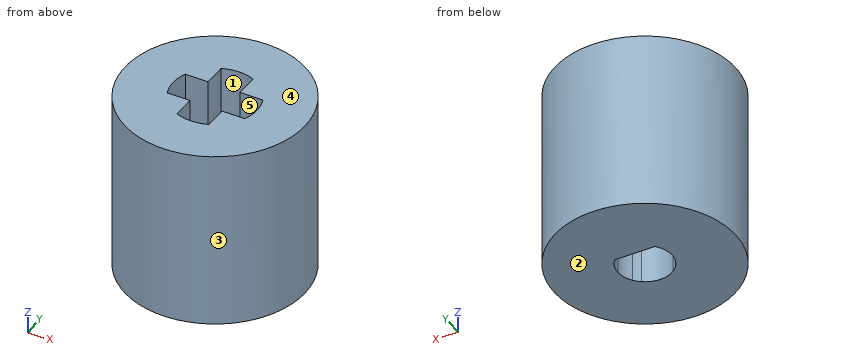
from build123d import *

# Parameters (mm, degrees)
SKETCH1_R           = 5
SKETCH1_R_2         = 2.34
BOSS_EXTRUDE1_DEPTH = 5
BOSS_EXTRUDE2_START = -5
SKETCH1_3_R         = 5
SKETCH1_3_R_2       = 2.34
BOSS_EXTRUDE2_DEPTH = 5


with BuildPart() as part:
    # Sketch1 → Boss-Extrude1 (new body)
    # profile 1 of 11: a face of its own
    with BuildSketch(Plane.XY):
        Circle(SKETCH1_R)
        Circle(SKETCH1_R_2, mode=Mode.SUBTRACT)
    # profile 2 of 11: a face of its own
    with BuildSketch(Plane.XY):
        with BuildLine():
            Line((-0.89, 1.207435298), (-0.89, 2.164139552))
            ThreePointArc((-0.89, 2.164139552), (-1.654629868, 1.654629868), (-2.164139552, 0.89))
            Line((-2.164139552, 0.89), (-1.207435298, 0.89))
            ThreePointArc((-1.207435298, 0.89), (-1.164034729, 0.946056631), (-1.118033989, 1))
            ThreePointArc((-1.118033989, 1), (-1.009359934, 1.109591152), (-0.89, 1.207435298))
        make_face()
    # profile 3 of 11: a face of its own
    with BuildSketch(Plane.XY):
        with BuildLine():
            ThreePointArc((2.164139552, 0.89), (1.654629868, 1.654629868), (0.89, 2.164139552))
            Line((0.89, 2.164139552), (0.89, 1.207435298))
            ThreePointArc((0.89, 1.207435298), (1.009359934, 1.109591152), (1.118033989, 1))
            ThreePointArc((1.118033989, 1), (1.164034729, 0.946056631), (1.207435298, 0.89))
            Line((1.207435298, 0.89), (2.164139552, 0.89))
        make_face()
    # profile 4 of 11: a face of its own
    with BuildSketch(Plane.XY):
        with BuildLine():
            Line((-0.89, 0.89), (-0.89, 1))
            Line((-0.89, 1), (-1.118033989, 1))
            ThreePointArc((-1.118033989, 1), (-1.164034729, 0.946056631), (-1.207435298, 0.89))
            Line((-1.207435298, 0.89), (-0.89, 0.89))
        make_face()
    # profile 5 of 11: a face of its own
    with BuildSketch(Plane.XY):
        with BuildLine():
            Line((-0.89, 1), (-0.89, 1.207435298))
            ThreePointArc((-0.89, 1.207435298), (-1.009359934, 1.109591152), (-1.118033989, 1))
            Line((-1.118033989, 1), (-0.89, 1))
        make_face()
    # profile 6 of 11: a face of its own
    with BuildSketch(Plane.XY):
        with BuildLine():
            ThreePointArc((1.118033989, 1), (1.009359934, 1.109591152), (0.89, 1.207435298))
            Line((0.89, 1.207435298), (0.89, 1))
            Line((0.89, 1), (1.118033989, 1))
        make_face()
    # profile 7 of 11: a face of its own
    with BuildSketch(Plane.XY):
        with BuildLine():
            Line((1.118033989, 1), (0.89, 1))
            Line((0.89, 1), (0.89, 0.89))
            Line((0.89, 0.89), (1.207435298, 0.89))
            ThreePointArc((1.207435298, 0.89), (1.164034729, 0.946056631), (1.118033989, 1))
        make_face()
    # profile 8 of 11: a face of its own
    with BuildSketch(Plane.XY):
        with BuildLine():
            Line((1.207435298, -0.89), (0.89, -0.89))
            Line((0.89, -0.89), (0.89, -1.207435298))
            ThreePointArc((0.89, -1.207435298), (1.060660172, -1.060660172), (1.207435298, -0.89))
        make_face()
    # profile 9 of 11: a face of its own
    with BuildSketch(Plane.XY):
        with BuildLine():
            ThreePointArc((0.89, -2.164139552), (1.654629868, -1.654629868), (2.164139552, -0.89))
            Line((2.164139552, -0.89), (1.207435298, -0.89))
            ThreePointArc((1.207435298, -0.89), (1.060660172, -1.060660172), (0.89, -1.207435298))
            Line((0.89, -1.207435298), (0.89, -2.164139552))
        make_face()
    # profile 10 of 11: a face of its own
    with BuildSketch(Plane.XY):
        with BuildLine():
            Line((-1.207435298, -0.89), (-2.164139552, -0.89))
            ThreePointArc((-2.164139552, -0.89), (-1.654629868, -1.654629868), (-0.89, -2.164139552))
            Line((-0.89, -2.164139552), (-0.89, -1.207435298))
            ThreePointArc((-0.89, -1.207435298), (-1.060660172, -1.060660172), (-1.207435298, -0.89))
        make_face()
    # profile 11 of 11: a face of its own
    with BuildSketch(Plane.XY):
        with BuildLine():
            Line((-0.89, -0.89), (-1.207435298, -0.89))
            ThreePointArc((-1.207435298, -0.89), (-1.060660172, -1.060660172), (-0.89, -1.207435298))
            Line((-0.89, -1.207435298), (-0.89, -0.89))
        make_face()
    extrude(amount=BOSS_EXTRUDE1_DEPTH)

    # Sketch1_3 → Boss-Extrude2 (add)
    # profile 1 of 16: a face of its own
    with BuildSketch(Plane.XY.offset(BOSS_EXTRUDE2_START)):
        Circle(SKETCH1_3_R)
        Circle(SKETCH1_3_R_2, mode=Mode.SUBTRACT)
    # profile 2 of 16: a face of its own
    with BuildSketch(Plane.XY.offset(BOSS_EXTRUDE2_START)):
        with BuildLine():
            ThreePointArc((0.89, -2.164139552), (1.654629868, -1.654629868), (2.164139552, -0.89))
            Line((2.164139552, -0.89), (1.207435298, -0.89))
            ThreePointArc((1.207435298, -0.89), (1.060660172, -1.060660172), (0.89, -1.207435298))
            Line((0.89, -1.207435298), (0.89, -2.164139552))
        make_face()
    # profile 3 of 16: a face of its own
    with BuildSketch(Plane.XY.offset(BOSS_EXTRUDE2_START)):
        with BuildLine():
            Line((-1.207435298, 0.89), (-2.164139552, 0.89))
            ThreePointArc((-2.164139552, 0.89), (-2.34, 0), (-2.164139552, -0.89))
            Line((-2.164139552, -0.89), (-1.207435298, -0.89))
            ThreePointArc((-1.207435298, -0.89), (-1.5, 0), (-1.207435298, 0.89))
        make_face()
    # profile 4 of 16: a face of its own
    with BuildSketch(Plane.XY.offset(BOSS_EXTRUDE2_START)):
        with BuildLine():
            ThreePointArc((2.34, 0), (2.295613921, 0.453604149), (2.164139552, 0.89))
            Line((2.164139552, 0.89), (1.207435298, 0.89))
            ThreePointArc((1.207435298, 0.89), (1.424982973, 0.46842665), (1.5, 0))
            ThreePointArc((1.5, 0), (1.424982973, -0.46842665), (1.207435298, -0.89))
            Line((1.207435298, -0.89), (2.164139552, -0.89))
            ThreePointArc((2.164139552, -0.89), (2.295613921, -0.453604149), (2.34, 0))
        make_face()
    # profile 5 of 16: a face of its own
    with BuildSketch(Plane.XY.offset(BOSS_EXTRUDE2_START)):
        with BuildLine():
            ThreePointArc((2.164139552, 0.89), (1.654629868, 1.654629868), (0.89, 2.164139552))
            Line((0.89, 2.164139552), (0.89, 1.207435298))
            ThreePointArc((0.89, 1.207435298), (1.009359934, 1.109591152), (1.118033989, 1))
            ThreePointArc((1.118033989, 1), (1.164034729, 0.946056631), (1.207435298, 0.89))
            Line((1.207435298, 0.89), (2.164139552, 0.89))
        make_face()
    # profile 6 of 16: a face of its own
    with BuildSketch(Plane.XY.offset(BOSS_EXTRUDE2_START)):
        with BuildLine():
            ThreePointArc((0.89, 2.164139552), (0, 2.34), (-0.89, 2.164139552))
            Line((-0.89, 2.164139552), (-0.89, 1.207435298))
            ThreePointArc((-0.89, 1.207435298), (0, 1.5), (0.89, 1.207435298))
            Line((0.89, 1.207435298), (0.89, 2.164139552))
        make_face()
    # profile 7 of 16: a face of its own
    with BuildSketch(Plane.XY.offset(BOSS_EXTRUDE2_START)):
        with BuildLine():
            Line((-0.89, -1.207435298), (-0.89, -2.164139552))
            ThreePointArc((-0.89, -2.164139552), (0, -2.34), (0.89, -2.164139552))
            Line((0.89, -2.164139552), (0.89, -1.207435298))
            ThreePointArc((0.89, -1.207435298), (0, -1.5), (-0.89, -1.207435298))
        make_face()
    # profile 8 of 16: a face of its own
    with BuildSketch(Plane.XY.offset(BOSS_EXTRUDE2_START)):
        with BuildLine():
            Line((-0.89, 1.207435298), (-0.89, 2.164139552))
            ThreePointArc((-0.89, 2.164139552), (-1.654629868, 1.654629868), (-2.164139552, 0.89))
            Line((-2.164139552, 0.89), (-1.207435298, 0.89))
            ThreePointArc((-1.207435298, 0.89), (-1.164034729, 0.946056631), (-1.118033989, 1))
            ThreePointArc((-1.118033989, 1), (-1.009359934, 1.109591152), (-0.89, 1.207435298))
        make_face()
    # profile 9 of 16: a face of its own
    with BuildSketch(Plane.XY.offset(BOSS_EXTRUDE2_START)):
        with BuildLine():
            Line((-1.207435298, 0.89), (-2.164139552, 0.89))
            ThreePointArc((-2.164139552, 0.89), (-2.34, 0), (-2.164139552, -0.89))
            Line((-2.164139552, -0.89), (-1.207435298, -0.89))
            ThreePointArc((-1.207435298, -0.89), (-1.5, 0), (-1.207435298, 0.89))
        make_face()
    # profile 10 of 16: a face of its own
    with BuildSketch(Plane.XY.offset(BOSS_EXTRUDE2_START)):
        with BuildLine():
            ThreePointArc((2.34, 0), (2.295613921, 0.453604149), (2.164139552, 0.89))
            Line((2.164139552, 0.89), (1.207435298, 0.89))
            ThreePointArc((1.207435298, 0.89), (1.424982973, 0.46842665), (1.5, 0))
            ThreePointArc((1.5, 0), (1.424982973, -0.46842665), (1.207435298, -0.89))
            Line((1.207435298, -0.89), (2.164139552, -0.89))
            ThreePointArc((2.164139552, -0.89), (2.295613921, -0.453604149), (2.34, 0))
        make_face()
    # profile 11 of 16: a face of its own
    with BuildSketch(Plane.XY.offset(BOSS_EXTRUDE2_START)):
        with BuildLine():
            Line((-1.207435298, -0.89), (-2.164139552, -0.89))
            ThreePointArc((-2.164139552, -0.89), (-1.654629868, -1.654629868), (-0.89, -2.164139552))
            Line((-0.89, -2.164139552), (-0.89, -1.207435298))
            ThreePointArc((-0.89, -1.207435298), (-1.060660172, -1.060660172), (-1.207435298, -0.89))
        make_face()
    # profile 12 of 16: a face of its own
    with BuildSketch(Plane.XY.offset(BOSS_EXTRUDE2_START)):
        with BuildLine():
            ThreePointArc((1.118033989, 1), (1.009359934, 1.109591152), (0.89, 1.207435298))
            Line((0.89, 1.207435298), (0.89, 1))
            Line((0.89, 1), (1.118033989, 1))
        make_face()
    # profile 13 of 16: a face of its own
    with BuildSketch(Plane.XY.offset(BOSS_EXTRUDE2_START)):
        with BuildLine():
            ThreePointArc((0.89, 1.207435298), (0, 1.5), (-0.89, 1.207435298))
            Line((-0.89, 1.207435298), (-0.89, 1))
            Line((-0.89, 1), (0.89, 1))
            Line((0.89, 1), (0.89, 1.207435298))
        make_face()
    # profile 14 of 16: a face of its own
    with BuildSketch(Plane.XY.offset(BOSS_EXTRUDE2_START)):
        with BuildLine():
            Line((-0.89, 1), (-0.89, 1.207435298))
            ThreePointArc((-0.89, 1.207435298), (-1.009359934, 1.109591152), (-1.118033989, 1))
            Line((-1.118033989, 1), (-0.89, 1))
        make_face()
    # profile 15 of 16: a face of its own
    with BuildSketch(Plane.XY.offset(BOSS_EXTRUDE2_START)):
        with BuildLine():
            ThreePointArc((0.89, 2.164139552), (0, 2.34), (-0.89, 2.164139552))
            Line((-0.89, 2.164139552), (-0.89, 1.207435298))
            ThreePointArc((-0.89, 1.207435298), (0, 1.5), (0.89, 1.207435298))
            Line((0.89, 1.207435298), (0.89, 2.164139552))
        make_face()
    # profile 16 of 16: a face of its own
    with BuildSketch(Plane.XY.offset(BOSS_EXTRUDE2_START)):
        with BuildLine():
            Line((-0.89, -1.207435298), (-0.89, -2.164139552))
            ThreePointArc((-0.89, -2.164139552), (0, -2.34), (0.89, -2.164139552))
            Line((0.89, -2.164139552), (0.89, -1.207435298))
            ThreePointArc((0.89, -1.207435298), (0, -1.5), (-0.89, -1.207435298))
        make_face()
    extrude(amount=BOSS_EXTRUDE2_DEPTH)


solid = part.part
Could you check a few things on this model? Use its own coordinates, in mm. Face numbers are marked on the shaded views. A direction names the side the tool comes from. Give positions to 0.01 mm unless a question says otherwise; leave off trailing zeros. Order: outer loops, then holes, each group sorted by start corner. A loop starts at its lowest first (then second) coordinate and runs counter-clockwise, first axis right, second up.
Item 1: If we section it at A-A, the plane x = 0: Write out the boundary of the cut face in (y, z), plus the area to 3 significant figures.
Item 2: I need wall thicknesses on line 1 (X direction, y = -1.75, z = 2.25); line 2 (Y direction, x = -0.75, z = -0.5); line 3 (Y direction, x = -2, z = 4.25). Which ranges of each line are inside material? Lowest first, please.
Item 3: For the marked faces 1 and 2, which set-ups out of +Z, -Z, +X, -X, +Y, -Y let a thin tool reach every point of the face, with its end or its side?
Item 4: If we mould it in two halves opening along Y, with no side actions, what happens to the marked faces 3, 4 and 5? For each: pulls with the +Y half, pulls with the -Y half, needs draft (parallel to the pull), parting line crosses it, or undercut.
Item 5: If we section it at C-C, the plane y = 0.75: Write out the boundary of the cut face in (x, z), plus the area to 3 significant figures.
Item 6: If we section it at D-D, the plane x = 1.75: Write out the boundary of the cut face in (y, z).
Item 7: I'm going to push flat-ended pins straight in: pin 1 (1.4 mm diameter, centred on x = -1, z = 3, fed in from -Y); pin 2 (6 mm diameter, centred on x = -3.5, z = -1.5, fed in from +Y); pin 3 (0.6 mm diameter, centred on x = 2, y = 0, fed in from +Z). Where does each tip first touch, or does it pass through?
Item 8: If we section it at B-B, the plane z = 0.75: Write out the boundary of the cut face in (x, y), plus the area to 3 significant figures.
Values:
1. outline: (-5, -5) - (-1.5, -5) - (-1.5, 0) - (-2.34, 0) - (-2.34, 5) - (-5, 5) - close; (1, -5) - (5, -5) - (5, 5) - (2.34, 5) - (2.34, 0) - (1, 0) - close
1. area: 64.1 mm2
2. line 1: x = -4.68 to -0.89, 0.89 to 4.68
2. line 2: y = -4.94 to -1.3, 1 to 4.94
2. line 3: y = -4.58 to -0.89, 0.89 to 4.58
3. face 1: +Z
3. face 2: -Z, +X, -X, +Y, -Y
4. face 3: parting line crosses it
4. face 4: needs draft
4. face 5: undercut
5. outline: (-4.94, -5) - (-1.3, -5) - (-1.3, 0) - (-2.22, 0) - (-2.22, 5) - (-4.94, 5) - close; (1.3, -5) - (4.94, -5) - (4.94, 5) - (2.22, 5) - (2.22, 0) - (1.3, 0) - close
5. area: 63.7 mm2
6. outline: (-4.68, -5) - (4.68, -5) - (4.68, 5) - (0.89, 5) - (0.89, 0) - (-0.89, 0) - (-0.89, 5) - (-4.68, 5) - close
7. pin 1: stops at y = -4.99
7. pin 2: stops at y = 4.97
7. pin 3: stops at z = 0
8. outline: circle Ø10 at (0, 0); hole (-2.16, -0.89) - (-0.89, -0.89) - (-0.89, -2.16) arc R2.34 ccw to (0.89, -2.16) - (0.89, -0.89) - (2.16, -0.89) arc R2.34 ccw to (2.16, 0.89) - (0.89, 0.89) - (0.89, 2.16) arc R2.34 ccw to (-0.89, 2.16) - (-0.89, 0.89) - (-2.16, 0.89) arc R2.34 ccw to start
8. area: 65.5 mm2
